from build123d import *

# Parameters (mm, degrees)
F0_W     = 180
F0_H     = 140
F1_DEPTH = 2.5
F2_R     = 1.5
F3_DEPTH = 5
F4_R     = 10


with BuildPart() as f1:
    # F0 (on Front) → F1 (new body)
    with BuildSketch(Plane.XZ):
        Rectangle(F0_W, F0_H)
    extrude(amount=F1_DEPTH)

    # F2 (on face) → F3 (cut)
    with BuildSketch(Plane.XZ.offset(2.5)):
        with Locations((75.857864, 55.857864)):
            Circle(F2_R)
        with Locations((-75.857864, 55.857864)):
            Circle(F2_R)
        with Locations((75.857864, -55.857864)):
            Circle(F2_R)
        with Locations((-75.857864, -55.857864)):
            Circle(F2_R)
        with BuildLine():
            ThreePointArc((29, -63), (28.707107, -62.292893), (28, -62))
            ThreePointArc((28, -62), (27.292893, -63.707107), (29, -63))
        make_face()
        with BuildLine():
            ThreePointArc((29, -27), (28, -26), (27, -27))
            Line((27, -27), (28, -27))
            Line((28, -27), (28, -28))
            ThreePointArc((28, -28), (28.707107, -27.707107), (29, -27))
        make_face()
        with BuildLine():
            Line((28, -27), (27, -27))
            ThreePointArc((27, -27), (27.292893, -27.707107), (28, -28))
            Line((28, -28), (28, -27))
        make_face()
        with BuildLine():
            ThreePointArc((-27, -63), (-27.292893, -62.292893), (-28, -62))
            Line((-28, -62), (-28, -63))
            Line((-28, -63), (-28, -64))
            ThreePointArc((-28, -64), (-27.292893, -63.707107), (-27, -63))
        make_face()
        with BuildLine():
            Line((-28, -63), (-28, -62))
            ThreePointArc((-28, -62), (-29, -63), (-28, -64))
            Line((-28, -64), (-28, -63))
        make_face()
        with BuildLine():
            ThreePointArc((-28, -28), (-27.292893, -27.707107), (-27, -27))
            Line((-27, -27), (-28, -27))
            Line((-28, -27), (-28, -28))
        make_face()
        with BuildLine():
            Line((-28, -27), (-27, -27))
            ThreePointArc((-27, -27), (-28.707107, -26.292893), (-28, -28))
            Line((-28, -28), (-28, -27))
        make_face()
        with BuildLine():
            Line((-8.75, 20), (-8.75, 0))
            Line((-8.75, 0), (-8.75, -20))
            ThreePointArc((-8.75, -20), (-7.826238, -23.913119), (-5.25, -27))
            Line((-5.25, -27), (5.25, -27))
            ThreePointArc((5.25, -27), (7.826238, -23.913119), (8.75, -20))
            Line((8.75, -20), (8.75, 0))
            Line((8.75, 0), (8.75, 20))
            ThreePointArc((8.75, 20), (0, 28.75), (-8.75, 20))
        make_face()
        with BuildLine():
            Line((5.25, -27), (-5.25, -27))
            ThreePointArc((-5.25, -27), (0, -28.75), (5.25, -27))
        make_face()
        with Locations((-60.1, 52.1)):
            Circle(F2_R)
        with BuildLine():
            ThreePointArc((-10.4, 50.8), (-11.149166, 52.098556), (-12.648331, 52.1))
            ThreePointArc((-12.648331, 52.1), (-12.650834, 49.501444), (-10.4, 50.8))
        make_face()
        with BuildLine():
            ThreePointArc((-25.6, 0), (-27.1, 1.5), (-28.6, 0))
            ThreePointArc((-28.6, 0), (-27.1, -1.5), (-25.6, 0))
        make_face()
        with BuildLine():
            ThreePointArc((-55, 1.5), (-56.06066, 1.06066), (-56.5, 0))
            Line((-56.5, 0), (-55, 0))
            Line((-55, 0), (-55, 1.5))
        make_face()
        with BuildLine():
            Line((-55, 0), (-56.5, 0))
            ThreePointArc((-56.5, 0), (-55, -1.5), (-53.5, 0))
            Line((-53.5, 0), (-55, 0))
        make_face()
        with Locations((-86, 33.5)):
            Circle(F2_R)
        with BuildLine():
            ThreePointArc((-68.5, 33.5), (-70, 35), (-71.5, 33.5))
            ThreePointArc((-71.5, 33.5), (-70, 32), (-68.5, 33.5))
        make_face()
        with BuildLine():
            ThreePointArc((-68.5, -33.5), (-70, -32), (-71.5, -33.5))
            ThreePointArc((-71.5, -33.5), (-70, -35), (-68.5, -33.5))
        make_face()
        with Locations((-86, -33.5)):
            Circle(F2_R)
        with BuildLine():
            Line((-55, 1.5), (-55, 0))
            Line((-55, 0), (-53.5, 0))
            ThreePointArc((-53.5, 0), (-53.93934, 1.06066), (-55, 1.5))
        make_face()
        with BuildLine():
            ThreePointArc((15.5, 0), (15.06066, 1.06066), (14, 1.5))
            ThreePointArc((14, 1.5), (12.93934, -1.06066), (15.5, 0))
        make_face()
        with BuildLine():
            ThreePointArc((14, 56.5), (15.06066, 56.93934), (15.5, 58))
            Line((15.5, 58), (14, 58))
            Line((14, 58), (14, 56.5))
        make_face()
        with BuildLine():
            Line((14, 58), (15.5, 58))
            ThreePointArc((15.5, 58), (12.93934, 59.06066), (14, 56.5))
            Line((14, 56.5), (14, 58))
        make_face()
        with BuildLine():
            ThreePointArc((61.5, 58), (61.93934, 56.93934), (63, 56.5))
            Line((63, 56.5), (63, 58))
            Line((63, 58), (61.5, 58))
        make_face()
        with BuildLine():
            Line((63, 58), (63, 56.5))
            ThreePointArc((63, 56.5), (64.06066, 56.93934), (64.5, 58))
            ThreePointArc((64.5, 58), (63, 59.5), (61.5, 58))
            Line((61.5, 58), (63, 58))
        make_face()
        with BuildLine():
            ThreePointArc((63, 1.5), (61.93934, -1.06066), (64.5, 0))
            Line((64.5, 0), (63, 0))
            Line((63, 0), (63, 1.5))
        make_face()
        with BuildLine():
            Line((63, 0), (64.5, 0))
            ThreePointArc((64.5, 0), (64.06066, 1.06066), (63, 1.5))
            Line((63, 1.5), (63, 0))
        make_face()
        with Locations((70, 33.5)):
            Circle(F2_R)
        with BuildLine():
            ThreePointArc((87.5, 33.5), (86, 35), (84.5, 33.5))
            ThreePointArc((84.5, 33.5), (86, 32), (87.5, 33.5))
        make_face()
        with BuildLine():
            ThreePointArc((87.5, -33.5), (86, -32), (84.5, -33.5))
            ThreePointArc((84.5, -33.5), (86, -35), (87.5, -33.5))
        make_face()
        with Locations((70, -33.5)):
            Circle(F2_R)
    extrude(amount=-F3_DEPTH, mode=Mode.SUBTRACT)

    # F4
    f4_edges = [f1.edges().sort_by_distance(p)[0] for p in [
        (-90, -1.25, 70),
        (-90, -1.25, -70),
        (90, -1.25, -70),
        (90, -1.25, 70),
    ]]
    fillet(f4_edges, radius=F4_R)


solid = f1.part
Work out the finished part from the listing and answer in its coordinate system (mm). A direction names the side the tool comes from. Give positions to 0.01 mm unless a question says otherwise; leave off trailing zeros. Write each loop counter-clockwise with the first axis right and the second up, starting at its lowest first coordinate (ties: lowest second). Pieces come first, ordered by that corner, then holes.
Q1. The part is cut by section A-A on z = -17. Give the vertices of the cut face in (x, y).
Answer:
outline: (-90, -2.5) - (-8.75, -2.5) - (-8.75, 0) - (-90, 0) - close; (8.75, -2.5) - (90, -2.5) - (90, 0) - (8.75, 0) - close
Q2. Straight lines are drawn through the part: L1, parallel to Z at x = -70, y = -0.8; L2, parallel to Z at x = 63, y = -1.9; L3, parallel to X at y = -0.7, z = -27. For each, find the intervals that lie inside material, in ascending order.
Answer:
L1: z = -70 to -35, -32 to 32, 35 to 70
L2: z = -70 to -1.5, 1.5 to 56.5, 59.5 to 70
L3: x = -90 to -29, -27 to -5.25, 5.25 to 27, 29 to 90
Q3. A tool of negligible diameter and unlimited length cuts with its end or side. For faces 1 (the face through (0.192, -1.268, 28.748)), 2 (the face through (19, 0, 1)), from which of +Z, -Z, +X, -X, +Y, -Y can it reach the whole face along a straight path? Write none if from no direction.
Answer:
face 1: +Y, -Y
face 2: +Z, -Z, +X, -X, +Y
Q4. The part is cut by section B-B on y = -1.2. State how many separate pieces and enclosed holes the cut face has, and give its area (3 significant figures).
Answer:
separate pieces: 1
enclosed holes: 25
area: 24,000 mm2
Q5. Given pin 1 (2.5 mm diameter, centred on x = 70, z = -33.5, fed in from -Y), flat-ended and moving along its own axis, determine where the tip first touches the part or whether it passes through.
Answer:
pin 1: passes through
